Geometry: final body of the model. Coordinates: model frame, mm. Give positions to 0.01 mm unless a question says otherwise; leave off trailing zeros. Write each loop counter-clockwise with the first axis right and the second up, starting at its lowest first coordinate (ties: lowest second). Pieces come first, ordered by that corner, then holes.
from build123d import *

# Parameters (mm, degrees)
SKETCH_1_W                = 6
SKETCH_1_H                = 21
HOLE_WIZARD_5_0_5_1_D     = 5
HOLE_WIZARD_5_0_5_2_D     = 5
HOLE_WIZARD_5_0_5_2_DEPTH = 18
SKETCH_5_W                = 2
SKETCH_5_H                = 4.5
HOLE_WIZARD_4_0_4_2_D     = 4


with BuildPart() as part:
    # 草图1 → 旋转1 (revolve)
    with BuildSketch(Plane.XZ.offset(40), mode=Mode.PRIVATE) as revolve_1_sk:
        with Locations((12, -20.5)):
            Rectangle(SKETCH_1_W, SKETCH_1_H)
    revolve(revolve_1_sk.sketch.rotate(Axis((9, -40, -10), (0, 0, -1)), 180), axis=Axis((9, -40, -10), (0, 0, -1)))

    # Ø5.0 (5) 直径孔1 (through all)
    with Locations(Plane(origin=(0, 0, -31), x_dir=(-1, 0, 0), z_dir=(0, 0, -1))):
        with Locations((-9, -40)):
            Hole(HOLE_WIZARD_5_0_5_1_D / 2)

    # Ø5.0 (5) 直径孔2
    with Locations(Plane(origin=(9, -46, -26), x_dir=(-1, 0, 0), z_dir=(0, -1, 0))):
        with Locations((0, 0)):
            Hole(HOLE_WIZARD_5_0_5_2_D / 2, depth=HOLE_WIZARD_5_0_5_2_DEPTH)

    # 草图5 → Ø4.0 (4) 直径孔1 (revolve, cut)
    with BuildSketch(Plane(origin=(9, -41.5, -14.5), x_dir=(0, 0, 1), z_dir=(1, 0, 0))):
        with Locations((1, 2.25)):
            Rectangle(SKETCH_5_W, SKETCH_5_H)
    revolve(axis=Axis((9, -35.15, -14.5), (0, -1, 0)), mode=Mode.SUBTRACT)

    # Ø4.0 (4) 直径孔2 (through all)
    with Locations(Plane(origin=(0, -38.5, 0), x_dir=(-1, 0, 0), z_dir=(0, -1, 0))):
        with Locations((-9, 14.5)):
            Hole(HOLE_WIZARD_4_0_4_2_D / 2)


solid = part.part
Q1. Section C-C on z = -22. Output: boundary loops of the cut face in (x, y).
Filled sheet:
outline: circle Ø12 at (9, -40); hole circle Ø5 at (9, -40)
Q2. Section D-D on z = -14.5. Output: boundary loops of the cut face in (x, y), plus the area to 3 significant figures.
Filled sheet:
outline: (7, -45.66) - (7, -41.5) arc R2.5 cw to (7, -38.5) - (7, -34.34) arc R6 ccw to start; (11, -45.66) arc R6 ccw to (11, -34.34) - (11, -38.5) arc R2.5 cw to (11, -41.5) - close
area: 64.0 mm2
Q3. Ray query, line 1 along Z through (x, y) = (9, -44.25); line 2 along Y through (x, z) = (9, -20.75); line 3 along Z through (x, y) = (10.25, -35). Return the intervals inside material, ascending.
Filled sheet:
line 1: z = -31 to -28.5, -23.5 to -16.5, -12.5 to -10
line 2: y = -46 to -42.5, -37.5 to -34
line 3: z = -31 to -28.17, -23.83 to -16.06, -12.94 to -10
Q4. Section B-B on y = -37. Output: boundary loops of the cut face in (x, z).
Filled sheet:
outline: (3.8, -31) - (14.2, -31) - (14.2, -10) - (3.8, -10) - close; hole circle Ø5 at (9, -26); hole circle Ø4 at (9, -14.5)
Q5. Pin query (flat end, axial travel): P1, Ø4.5, axis at x = 9, y = -40, coming from the +Z side; P2, Ø5, axis at x = 9, z = -14.5, coming from the +Y side; P3, Ø1, axis at x = 6, z = -12.5, coming from the -Y side; P4, Ø1, axis at x = 5.5, z = -24, coming from the +Y side. Return the tip coordinate at first contact, or that it passes through.
Filled sheet:
P1: passes through
P2: stops at y = -34
P3: stops at y = -45.45
P4: stops at y = -34.8
Q6. Section A-A on x = 9. Output: boundary loops of the cut face in (y, z), plus the area to 3 significant figures.
Filled sheet:
outline: (-46, -31) - (-42.5, -31) - (-42.5, -28.5) - (-46, -28.5) - close; (-46, -23.5) - (-42.5, -23.5) - (-42.5, -16.5) - (-46, -16.5) - close; (-46, -12.5) - (-42.5, -12.5) - (-42.5, -10) - (-46, -10) - close; (-37.5, -31) - (-34, -31) - (-34, -28.5) - (-37.5, -28.5) - close; (-37.5, -23.5) - (-34, -23.5) - (-34, -16.5) - (-37.5, -16.5) - close; (-37.5, -12.5) - (-34, -12.5) - (-34, -10) - (-37.5, -10) - close
area: 84.0 mm2
Q7. Pull-direction query (X, two-part tool) for faces 1 (the flat face through (12, -40, -31)), 2 (the cylindrical face through (7, -43.6, -24.5)), 3 (the cylindrical face through (11.385, -36.289, -26.751)), 4 (the cylindrical face through (3.46, -42.3, -20.35)); classes: released by +X, released by -X, zero draft, split by the parting line, or undercut.
Filled sheet:
face 1: zero draft
face 2: undercut
face 3: undercut
face 4: split by the parting line
